For this review, take the finished solid that the model builds, in its own axes (mm). Face numbers are marked on the shaded views. A direction names the side the tool comes from. Give positions to 0.01 mm unless a question says otherwise; leave off trailing zeros. Order: outer loops, then holes, each group sorted by start corner. A loop starts at its lowest first (then second) coordinate and runs counter-clockwise, first axis right, second up. Notation, with made-up numbers: (80, 69) - (109, 69) arc R21 cw to (109, 97) - close; hole circle Ø1 at (-7, 63). An arc over 180 degrees is marked (long way). Answer as a JSON object with one key per item and string values. Group by question number.
from build123d import *

# Parameters (mm, degrees)
F0_R     = 3.175
F0_W     = 31.75
F0_H     = 12.7
F1_DEPTH = 12.7
F2_DEPTH = 25.4
F3_DEPTH = 38.1
F0_W_2   = 12.7
F0_H_2   = 50.8
F4_DEPTH = 50.8
F6_DEPTH = 50.801
F8_DEPTH = 82.551


with BuildPart() as f1:
    # F0 (on Top) → F1 (new body)
    with BuildSketch(Plane.XY):
        with BuildLine():
            Line((12.7, -12.7), (12.7, -25.4))
            Line((12.7, -25.4), (25.4, -25.4))
            ThreePointArc((25.4, -25.4), (38.870384, -19.820384), (44.45, -6.35))
            Line((44.45, -6.35), (12.7, -6.35))
            Line((12.7, -6.35), (12.7, -12.7))
        make_face()
        with Locations((25.4, -12.7)):
            Circle(F0_R, mode=Mode.SUBTRACT)
        with Locations((28.575, 0)):
            Rectangle(F0_W, F0_H)
        with BuildLine():
            Line((25.4, 25.4), (12.7, 25.4))
            Line((12.7, 25.4), (12.7, 12.7))
            Line((12.7, 12.7), (12.7, 6.35))
            Line((12.7, 6.35), (44.45, 6.35))
            ThreePointArc((44.45, 6.35), (38.870384, 19.820384), (25.4, 25.4))
        make_face()
        with Locations((25.4, 12.7)):
            Circle(F0_R, mode=Mode.SUBTRACT)
    extrude(amount=F1_DEPTH)

    # F0 (on Top) → F2 (join)
    with BuildSketch(Plane.XY):
        Polygon((-12.7, -12.7), (-12.7, -25.4), (12.7, -25.4), (12.7, -12.7), (0, -12.7), align=None)
        Polygon((12.7, 25.4), (-12.7, 25.4), (-12.7, 12.7), (0, 12.7), (12.7, 12.7), align=None)
    extrude(amount=F2_DEPTH)

    # F0 (on Top) → F3 (join)
    with BuildSketch(Plane.XY):
        Polygon((12.7, 12.7), (0, 12.7), (0, -12.7), (12.7, -12.7), (12.7, -6.35), (12.7, 6.35), align=None)
    extrude(amount=F3_DEPTH)

    # F0 (on Top) → F4 (join)
    with BuildSketch(Plane.XY):
        with Locations((-31.75, 0)):
            Rectangle(F0_W_2, F0_H_2)
        Polygon((-12.7, 25.4), (-25.4, 25.4), (-25.4, -25.4), (-12.7, -25.4), (-12.7, -12.7), (0, -12.7), (0, 12.7), (-12.7, 12.7), align=None)
    extrude(amount=F4_DEPTH)

    # F5 (on face) → F6 (cut, through all)
    with BuildSketch(Plane.XZ.offset(25.4)):
        Polygon((-25.4, 50.8), (-38.1, 50.8), (-38.1, 38.1), align=None)
    extrude(amount=-F6_DEPTH, mode=Mode.SUBTRACT)

    # F7 (on face) → F8 (cut, through all)
    with BuildSketch(Plane.YZ.offset(44.45)):
        with BuildLine():
            Line((-6.35, 12.7), (6.35, 12.7))
            ThreePointArc((6.35, 12.7), (0, 19.05), (-6.35, 12.7))
        make_face()
        with BuildLine():
            ThreePointArc((-6.35, 12.7), (0, 6.35), (6.35, 12.7))
            Line((6.35, 12.7), (-6.35, 12.7))
        make_face()
    extrude(amount=-F8_DEPTH, mode=Mode.SUBTRACT)


solid = f1.part
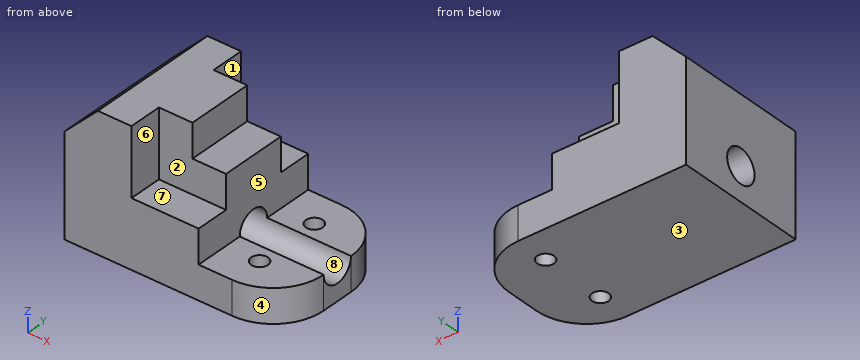
1) Consider section A-A (x = 10). Give the boundary of the cut face in (y, z).
2) Consider section C-C (y = -2). Give the boundary of the cut face in (x, z), plus the area to 3 significant figures.
3) Mouldability with a two-part tool opening along Z and no side actions: class the marked faces 6, 7 and 8 as released by +Z, released by -Z, zero draft, split by the parting line, or undercut.
4) For the marked faces 1, 2, 3, 4 and 5, list the 3-axis set-ups (+Z, -Z, +X, -X, +Y, -Y) from which the entire face can be reached by the end or side of a thin tool; tool diameter is ignored.
5) For line 1 (Z direction, x = 9, y = 0); line 2 (Y direction, x = 25, z = 7); line 3 (Y direction, x = -0.5, z = 37.5), list the stretches that pass through material, from the lowest coordinate up.
6) Consider section D-D (z = 10). Give the boundary of the cut face in (x, y) (3 decimals), plus the area to 3 significant figures.
7) For pin 1 (6 mm diameter, centred on x = 3.5, y = -19.5, fed in from -Z); pin 2 (12.5 mm diameter, centred on y = -5, z = 31, fed in from +X); pin 3 (7.5 mm diameter, centred on x = 25.4, y = 12.7, fed in from +Z); pin 4 (10 mm diameter, centred on y = -2, z = 45.5, fed in from +X), all flat-tipped, find the tip position at first contact; note any pin that passes through.
8) Consider section B-B (z = 28). Give the boundary of the cut face in (x, y), plus the area to 3 significant figures.
Result set:
{
 "1": {"outline": "(-25.4, 0) - (25.4, 0) - (25.4, 25.4) - (12.7, 25.4) - (12.7, 38.1) - (-12.7, 38.1) - (-12.7, 25.4) - (-25.4, 25.4) - close; hole circle Ø12.7 at (0, 12.7)"},
 "2": {"outline": "(-38.1, 0) - (44.45, 0) - (44.45, 6.67) - (-38.1, 6.67) - close; (-38.1, 18.73) - (12.7, 18.73) - (12.7, 38.1) - (0, 38.1) - (0, 50.8) - (-25.4, 50.8) - (-38.1, 38.1) - close", "area": "1,940 mm2"},
 "3": {"face 6": "zero draft", "face 7": "released by +Z", "face 8": "undercut"},
 "4": {"face 1": "+Z, +X, +Y", "face 2": "+Z, +X, -Y", "face 3": "-Z, +X, -X, +Y, -Y", "face 4": "+Z, -Z, +X, -Y", "face 5": "+Z, +X, +Y, -Y"},
 "5": {"line 1": "z = 0 to 6.35, 19.05 to 38.1", "line 2": "y = -25.4 to -15.85, -9.55 to -2.8, 2.8 to 9.55, 15.85 to 25.4", "line 3": "y = -12.7 to 12.7"},
 "6": {"outline": "(-38.1, -25.4) - (25.4, -25.4) arc R19.05 ccw to (44.45, -6.35) - (44.45, -5.747) - (-38.1, -5.747) - close; (-38.1, 5.747) - (44.45, 5.747) - (44.45, 6.35) arc R19.05 ccw to (25.4, 25.4) - (-38.1, 25.4) - close; hole circle Ø6.35 at (25.4, -12.7); hole circle Ø6.35 at (25.4, 12.7)", "area": "3,030 mm2"},
 "7": {"pin 1": "stops at z = 0", "pin 2": "stops at x = 12.7", "pin 3": "stops at z = 12.7", "pin 4": "stops at x = 0"},
 "8": {"outline": "(-38.1, -25.4) - (-12.7, -25.4) - (-12.7, -12.7) - (12.7, -12.7) - (12.7, 12.7) - (-12.7, 12.7) - (-12.7, 25.4) - (-38.1, 25.4) - close", "area": "1,940 mm2"}
}
